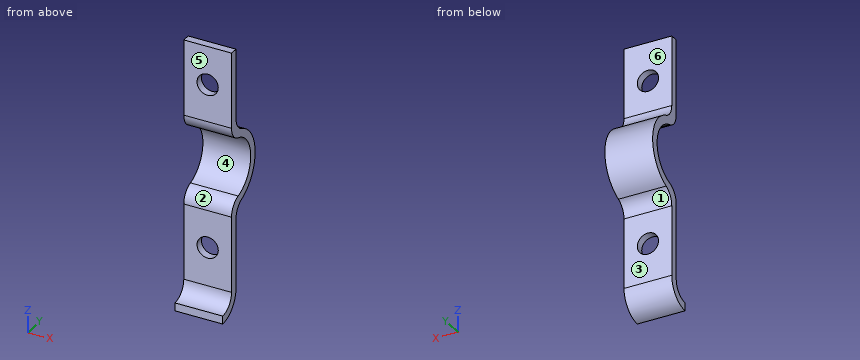
from build123d import *

# Parameters (mm, degrees)
BOSS_EXTRUDE1_DEPTH = 3.81
CUT_EXTRUDE1_REACH  = 5.81
SKETCH3_R           = 1.694754892


with BuildPart() as part:
    # Sketch2 → Boss-Extrude1 (new body, symmetric)
    with BuildSketch(Plane(origin=(0, 0, 0), x_dir=(0, 0, -1), z_dir=(1, 0, 0))):
        with BuildLine():
            Line((21.69668, -3.175), (22.96668, -3.175))
            ThreePointArc((22.96668, -3.175), (21.850756836, -0.480923164), (19.15668, 0.635))
            Line((19.15668, 0.635), (8.031181171, 0.635))
            ThreePointArc((8.031181171, 0.635), (6.602950056, 1.074581974), (5.669069062, 2.241176471))
            ThreePointArc((5.669069062, 2.241176471), (0, 6.096), (-5.669069062, 2.241176471))
            ThreePointArc((-5.669069062, 2.241176471), (-6.602950056, 1.074581974), (-8.031181171, 0.635))
            Line((-8.031181171, 0.635), (-19.15668, 0.635))
            Line((-19.15668, 0.635), (-19.15668, -0.635))
            Line((-19.15668, -0.635), (-7.115400973, -0.635))
            ThreePointArc((-7.115400973, -0.635), (-5.568940052, -0.109958714), (-4.66181443, 1.248103448))
            ThreePointArc((-4.66181443, 1.248103448), (0, 4.826), (4.66181443, 1.248103448))
            ThreePointArc((4.66181443, 1.248103448), (5.568940052, -0.109958714), (7.115400973, -0.635))
            Line((7.115400973, -0.635), (19.15668, -0.635))
            ThreePointArc((19.15668, -0.635), (20.952731224, -1.378948776), (21.69668, -3.175))
        make_face()
    extrude(amount=BOSS_EXTRUDE1_DEPTH, both=True)

    # Sketch3 → Cut-Extrude1 (cut, up to next)
    with BuildSketch(Plane(origin=(0, 0.635, 0), x_dir=(1, 0, 0), z_dir=(0, 1, 0)), mode=Mode.PRIVATE) as cut_extrude1_sk1:
        with Locations((0, 13.03528)):
            Circle(SKETCH3_R)
    cut_extrude1_tool1 = extrude(cut_extrude1_sk1.sketch, amount=-CUT_EXTRUDE1_REACH, mode=Mode.PRIVATE) & part.part
    add(cut_extrude1_tool1.solids().sort_by_distance((0, 0.635, -13.03528))[0], mode=Mode.SUBTRACT)
    # Sketch3 → Cut-Extrude1 (cut, up to next)
    with BuildSketch(Plane(origin=(0, 0.635, 0), x_dir=(1, 0, 0), z_dir=(0, 1, 0)), mode=Mode.PRIVATE) as cut_extrude1_sk2:
        with Locations((0, -13.03528)):
            Circle(SKETCH3_R)
    cut_extrude1_tool2 = extrude(cut_extrude1_sk2.sketch, amount=-CUT_EXTRUDE1_REACH, mode=Mode.PRIVATE) & part.part
    add(cut_extrude1_tool2.solids().sort_by_distance((0, 0.635, 13.03528))[0], mode=Mode.SUBTRACT)


solid = part.part
Geometry check sheet. Reference: the model listing, model coordinates, mm. Face numbers are marked on the shaded views. A direction names the side the tool comes from. Round coordinates to 2 decimals unless told otherwise and drop trailing zeros. Loops run counter-clockwise (first coordinate to the right, second up) from the corner with the lowest first, then second, coordinate; pieces in that order, holes last. Notation, with made-up numbers: (14.5, 50.5) - (67.5, 50.5) arc R24 ccw to (67.5, 79.5) - close; hole circle Ø10 at (-13, 7). An arc over 180 degrees is marked (long way). Answer as CSV lines item,"result".
(1) Material ranges on line 1 along Z through (x, y) = (0, -0.05); line 2 along Z through (x, y) = (0, -0.1); line 3 along Z through (x, y) = (-1.25, 1.25), recorded low to high.
Output values:
line 1,"z = -21.34 to -14.73, -11.34 to -5.49, 5.49 to 11.34, 14.73 to 19.16"
line 2,"z = -21.41 to -14.73, -11.34 to -5.56, 5.56 to 11.34, 14.73 to 19.16"
line 3,"z = -6.37 to -4.66, 4.66 to 6.37"
(2) Cross-section at D-D, the plane x = 2.5. Enter the section's corners in (y, z) (3 decimals).
Output values:
outline,"(-3.175, -22.967) arc R3.81 ccw to (0.635, -19.157) - (0.635, -8.031) arc R2.54 cw to (2.241, -5.669) arc R6.096 ccw to (2.241, 5.669) arc R2.54 cw to (0.635, 8.031) - (0.635, 19.157) - (-0.635, 19.157) - (-0.635, 7.115) arc R2.54 ccw to (1.248, 4.662) arc R4.826 cw to (1.248, -4.662) arc R2.54 ccw to (-0.635, -7.115) - (-0.635, -19.157) arc R2.54 cw to (-3.175, -21.697) - close"
(3) Depth check by flat-ended pin: pin 1 Ø2.5 at (x, z) = (0, 13.04) entering from -Y; pin 2 Ø1 at (x, y) = (3, 2.5) entering from -Z; pin 3 Ø4 at (x, z) = (0, -14) entering from -Y (3 decimals); pin 4 Ø1.5 at (x, y) = (1.5, 1) entering from -Z. Enter the tip coordinate at first touch or a pass-through.
Output values:
pin 1,"passes through"
pin 2,"stops at z = -5.78"
pin 3,"stops at y = -0.635"
pin 4,"stops at z = -20.83"
(4) Set-up check for the marked faces 4, 5 and 6: record each of +Z, -Z, +X, -X, +Y, -Y from which the full face is reachable in a straight line by a thin tool's end or side.
Output values:
face 4,"+X, -X, -Y"
face 5,"+Z, +X, -X, -Y"
face 6,"+Z, +X, -X, +Y"
(5) Release check for a two-part mould opening along Z. For the marked faces 1, 2 and 3 record: released by +Z, released by -Z, zero draft, split by the parting line, or undercut.
Output values:
face 1,"released by -Z"
face 2,"undercut"
face 3,"zero draft"
(6) Cross-section at A-A, the plane x = 0. Enter the section's corners in (y, z) (3 decimals), and give its area (3 significant figures).
Output values:
outline,"(-3.175, -22.967) arc R3.81 ccw to (0.635, -19.157) - (0.635, -14.73) - (-0.635, -14.73) - (-0.635, -19.157) arc R2.54 cw to (-3.175, -21.697) - close; (-0.635, -11.341) - (0.635, -11.341) - (0.635, -8.031) arc R2.54 cw to (2.241, -5.669) arc R6.096 ccw to (2.241, 5.669) arc R2.54 cw to (0.635, 8.031) - (0.635, 11.341) - (-0.635, 11.341) - (-0.635, 7.115) arc R2.54 ccw to (1.248, 4.662) arc R4.826 cw to (1.248, -4.662) arc R2.54 ccw to (-0.635, -7.115) - close; (-0.635, 14.73) - (0.635, 14.73) - (0.635, 19.157) - (-0.635, 19.157) - close"
area,"53.7 mm²"
(7) Cross-section at B-B, the plane y = 3. Enter the section's corners in (x, z), and give its area (3 significant figures).
Output values:
outline,"(-3.81, -5.31) - (3.81, -5.31) - (3.81, -3.78) - (-3.81, -3.78) - close; (-3.81, 3.78) - (3.81, 3.78) - (3.81, 5.31) - (-3.81, 5.31) - close"
area,"23.3 mm²"
(8) Cross-section at C-C, the plane z = 12. Enter the section's corners in (x, y) (3 decimals), and give its area (3 significant figures).
Output values:
outline,"(-3.81, -0.635) - (-1.342, -0.635) - (-1.342, 0.635) - (-3.81, 0.635) - close; (1.342, -0.635) - (3.81, -0.635) - (3.81, 0.635) - (1.342, 0.635) - close"
area,"6.27 mm²"
